Verification items for the finished model (mm, model axes). A direction names the side the tool comes from. Give positions to 0.01 mm unless a question says otherwise; leave off trailing zeros. Order: outer loops, then holes, each group sorted by start corner. A loop starts at its lowest first (then second) coordinate and runs counter-clockwise, first axis right, second up.
(1) Sectioned sample at A-A on z = 7.5. Record the cut outline in (x, y), plus the area to 3 significant figures.
(2) Gauge pin test, flat ends, axial feed: pin 1 (12 mm diameter, centred on y = -2.5, z = 11, fed in from +X); pin 2 (6 mm diameter, centred on x = 1, y = -1, fed in from +Z); pin 3 (1.5 mm diameter, centred on x = 6, z = 6.5, fed in from -Y). Record the tip position at first contact, or that the pin passes through.
(3) Mould release check, pull along Y, two halves, no side actions. Record for faces 1 (the face through (-6.269, 4.807, 17.135)), 2 (the face through (-6, 0, 11)), 3 (the face through (-2, -6, 20)): pulls with the +Y half, pulls with the -Y half, needs draft (parallel to the pull), parting line crosses it, or undercut.
(4) Access from +Z, -Z, +X, -X, +Y, -Y to the whole of each face (thin tool, end or side, straight path). Record for faces 4 (the face through (0, 0, -4)), 5 (the face through (-6.269, 4.807, 1.135)).
(5) Scan lines: L1, parallel to Y at x = 0, z = 7.75; L2, parallel to X at y = -4, z = 6.5; L3, parallel to X at y = -0.25, z = 3. Record each from-to range of solid material in increasing order.
```python
from build123d import *

# Parameters (mm, degrees)
LINEARPATTERN_COUNT = 10
LINEARPATTERN_PITCH = 2
SKETCH_R            = 7.9
PAD_DEPTH           = 20
SKETCH001_R         = 11
PAD001_DEPTH        = 4
FILLET_R            = 3
SKETCH002_R         = 6
POCKET_DEPTH        = 18
FILLET001_R         = 1


with BuildPart() as part:
    # Cone → Cone (revolve)
    with BuildSketch(Plane.XZ):
        Polygon((0, 0), (8.4, 0), (5, 2), (0, 2), align=None)
    cone = revolve(axis=Axis((0, 0, 0), (0, 0, 1)))

    # LinearPattern: Cone ×10
    with Locations(*[(0, 0, i * LINEARPATTERN_PITCH) for i in range(1, LINEARPATTERN_COUNT)]):
        add(cone)

    # Sketch (on Face21 of LinearPattern) → Pad (new body)
    with BuildSketch(Plane(origin=(0, 0, 0), x_dir=(1, 0, 0), z_dir=(0, 0, -1))):
        Circle(SKETCH_R)
    extrude(amount=-PAD_DEPTH)

    # Sketch001 (on Face33 of Pad) → Pad001 (join)
    with BuildSketch(Plane(origin=(0, 0, 0), x_dir=(1, 0, 0), z_dir=(0, 0, -1))):
        Circle(SKETCH001_R)
    extrude(amount=PAD001_DEPTH)

    # Fillet
    fillet_edges = [part.edges().sort_by_distance(p)[0] for p in [
        (-11, 0, -4),
    ]]
    fillet(fillet_edges, radius=FILLET_R)

    # Sketch002 (on Face34 of Fillet) → Pocket (cut)
    with BuildSketch(Plane.XY.offset(20)):
        Circle(SKETCH002_R)
    extrude(amount=-POCKET_DEPTH, mode=Mode.SUBTRACT)

    # Fillet001
    fillet001_edges = [part.edges().sort_by_distance(p)[0] for p in [
        (-7.9, 0, 20),
    ]]
    fillet(fillet001_edges, radius=FILLET001_R)


solid = part.part
```
Ans:
1. outline: circle Ø15.8 at (0, 0); hole circle Ø12 at (0, 0)
1. area: 83.0 mm2
2. pin 1: stops at x = 8.4
2. pin 2: stops at z = 2
2. pin 3: stops at y = -6.4
3. face 1: parting line crosses it
3. face 2: undercut
3. face 3: needs draft
4. face 4: -Z, +X, -X, +Y, -Y
4. face 5: none
5. L1: y = -7.9 to -6, 6 to 7.9
5. L2: x = -6.81 to -4.47, 4.47 to 6.81
5. L3: x = -7.9 to -5.99, 5.99 to 7.9
